Geometry check sheet. Reference: the model listing, model coordinates, mm. A direction names the side the tool comes from. Give positions to 0.01 mm unless a question says otherwise; leave off trailing zeros. Write each loop counter-clockwise with the first axis right and the second up, starting at its lowest first coordinate (ties: lowest second). Pieces come first, ordered by that corner, then holes. Notation, with made-up numbers: (65, 77) -> (75, 77) arc R15 cw to (75, 85) -> close; hole circle Ø9 at (-40, -5). An arc over 180 degrees is marked (long way). Write item = value, one per line. Start each with the question number.
1. Cross-section at D-D, the plane y = -33. Record the cut outline in (x, z), plus the area to 3 significant figures.
2. Set-up check for faces 4 (the cylindrical face through (-50.16, -125.472, 62.051)), 5 (the flat face through (32, -50.8, -25)), 6 (the flat face through (0, -89, 32)): record each of +Z, -Z, +X, -X, +Y, -Y from which the full face is reachable in a straight line by a thin tool's end or side.
3. Cross-section at B-B, the plane x = 8. Record the cut outline in (y, z), plus the area to 3 significant figures.
4. Mould release check, pull along X, two halves, no side actions. Record for faces 1 (the cylindrical face through (-100.072, -64.318, 62.051)), 2 (the cylindrical face through (-1.528, -125.551, 31.377)), 3 (the cylindrical face through (-62.684, -66.028, 0.889)): pulls with the +X half, pulls with the -X half, needs draft (parallel to the pull), parting line crosses it, or undercut.
5. Thickness scan on line 1 along Y through (x, z) = (-77.5, -38.5); line 2 along Z through (x, y) = (-11.5, -110.5); line 3 along Y through (x, z) = (56, 29). Record the ranges inside material, lowest first.
6. Depth check by flat-ended pin: P1, Ø16, axis at y = -73, z = -44, coming from the +X side; P2, Ø4, axis at x = 42, z = -10.5, coming from the -Y side; P3, Ø16, axis at y = -94.5, z = 43.5, coming from the +X side. Enter the tip coordinate at first touch or a pass-through.
7. Cross-section at C-C, the plane z = -52. Record the cut outline in (x, y).
8. Cross-section at A-A, the plane y = -101.5. Record the cut outline in (x, z).
```python
from build123d import *

# Parameters (mm, degrees)
F0_W     = 203.2
F0_H     = 127
F1_DEPTH = 127
F3_DEPTH = 76.2
F4_SIZE2 = 101.6
F4_SIZE  = 50.8
F5_R     = 5.08
F6_R     = 15.24
F7_DEPTH = 50.8
F8_R     = 15.301727391
F9_DEPTH = 127


with BuildPart() as f1:
    # F0 (on Front) → F1 (new body)
    with BuildSketch(Plane.XZ):
        Rectangle(F0_W, F0_H)
    extrude(amount=F1_DEPTH)

    # F2 (on face) → F3 (cut)
    with BuildSketch(Plane.XZ.offset(127)):
        Polygon((101.6, 63.5), (0, 63.5), (0, 0), (-35.2848060429, 0), (-35.2848060429, -63.5), (101.6, -63.5), align=None)
    extrude(amount=-F3_DEPTH, mode=Mode.SUBTRACT)

    # F4
    f4_edges = [f1.edges().sort_by_distance(p)[0] for p in [
        (101.6, -25.4, 63.5),
    ]]
    f4_side = f1.faces().sort_by_distance((-21.771429, -52.614286, 63.5))[0]
    chamfer(f4_edges, length=F4_SIZE, length2=F4_SIZE2, reference=f4_side)

    # F5
    f5_edges = [f1.edges().sort_by_distance(p)[0] for p in [
        (-50.8, -127, 63.5),
        (0, -88.9, 63.5),
        (76.2, -50.8, 12.7),
        (-101.6, -63.5, 63.5),
        (-25.4, 0, 63.5),
        (76.2, 0, 12.7),
        (-68.442403, -127, -63.5),
        (101.6, -25.4, -63.5),
        (50.8, -25.4, 63.5),
        (25.4, -50.8, 63.5),
        (0, -88.9, 0),
        (-35.284806, -88.9, -63.5),
        (-17.642403, -127, 0),
        (33.157597, -50.8, -63.5),
        (101.6, -25.4, -38.1),
        (-101.6, -63.5, -63.5),
        (101.6, 0, -50.8),
        (-17.642403, -50.8, 0),
        (0, -127, 31.75),
        (-35.284806, -127, -31.75),
        (0, 0, -63.5),
        (0, -50.8, 31.75),
        (-35.284806, -50.8, -31.75),
        (-101.6, -127, 0),
        (-101.6, 0, 0),
        (-35.284806, -88.9, 0),
        (101.6, -50.8, -50.8),
    ]]
    fillet(f5_edges, radius=F5_R)

    # F6 (on face) → F7 (cut, through all)
    with BuildSketch(Plane.XZ.offset(50.8)):
        with Locations((20.5951939571, -7.4171987902)):
            Circle(F6_R)
    extrude(amount=-F7_DEPTH, mode=Mode.SUBTRACT)

    # F8 (on face) → F9 (cut, through all)
    with BuildSketch(Plane.XY.offset(63.5)):
        with Locations((-76.8187716603, -60.167491436)):
            Circle(F8_R)
    extrude(amount=-F9_DEPTH, mode=Mode.SUBTRACT)


solid = f1.part
```
Answers:
q1.outline = (-101.6, -58.42) arc R5.08 ccw to (-96.52, -63.5) -> (96.52, -63.5) arc R5.08 ccw to (101.6, -58.42) -> (101.6, -39.3) arc R5.08 ccw to (101.06, -37.03) -> (52.2, 60.69) arc R5.08 ccw to (47.66, 63.5) -> (-96.52, 63.5) arc R5.08 ccw to (-101.6, 58.42) -> close; hole circle Ø30.48 at (20.6, -7.42)
q1.area = 22,500 mm^2
q2.face_4 = +Z, +X, -X, -Y
q2.face_5 = -Z, +X, -Y
q2.face_6 = +Z, -Z, +X, -Y
q3.outline = (-50.8, -58.42) arc R5.08 ccw to (-45.72, -63.5) -> (-5.08, -63.5) arc R5.08 ccw to (0, -58.42) -> (0, -16) -> (-50.8, -16) -> close; (-50.8, 1.16) -> (0, 1.16) -> (0, 58.42) arc R5.08 ccw to (-5.08, 63.5) -> (-45.72, 63.5) arc R5.08 ccw to (-50.8, 58.42) -> close
q3.area = 5,560 mm^2
q4.face_1 = pulls with the -X half
q4.face_2 = pulls with the +X half
q4.face_3 = undercut
q5.line_1 = -127 to -75.45, -44.88 to 0
q5.line_2 = 0 to 63.5
q5.line_3 = -50.8 to 0
q6.P1 = -35.28
q6.P2 = -50.8
q6.P3 = 0
q7.outline = (-101.6, -121.92) arc R5.08 ccw to (-96.52, -127) -> (-40.36, -127) arc R5.08 ccw to (-35.28, -121.92) -> (-35.28, -55.88) arc R5.08 cw to (-30.2, -50.8) -> (96.52, -50.8) arc R5.08 ccw to (101.6, -45.72) -> (101.6, -5.08) arc R5.08 ccw to (96.52, 0) -> (-96.52, 0) arc R5.08 ccw to (-101.6, -5.08) -> close; hole circle Ø30.6 at (-76.82, -60.17)
q8.outline = (-101.6, -58.42) arc R5.08 ccw to (-96.52, -63.5) -> (-40.36, -63.5) arc R5.08 ccw to (-35.28, -58.42) -> (-35.28, -5.08) arc R5.08 cw to (-30.2, 0) -> (-5.08, 0) arc R5.08 ccw to (0, 5.08) -> (0, 58.42) arc R5.08 ccw to (-5.08, 63.5) -> (-96.52, 63.5) arc R5.08 ccw to (-101.6, 58.42) -> close
